from build123d import *

# Parameters (mm, degrees)
SALIENTE_EXTRUIR1_DEPTH = 5
CROQUIS4_R              = 3.275
CORTAR_EXTRUIR3_DEPTH   = 15
CROQUIS5_R              = 1.5
CORTAR_EXTRUIR4_DEPTH   = 10


with BuildPart() as part:
    # Croquis1 → Saliente-Extruir1 (new, symmetric)
    with BuildSketch(Plane.XY):
        Polygon((3, -8.75), (3, 13.75), (0, 13.75), (0, -13.75), (10, -13.75), (10, -8.75), align=None)
        Polygon((0, -13.75), (0, 13.75), (-3, 13.75), (-3, -8.75), (-10, -8.75), (-10, -13.75), align=None)
    extrude(amount=SALIENTE_EXTRUIR1_DEPTH, both=True)

    # Croquis4 → Cortar-Extruir3 (cut)
    with BuildSketch(Plane(origin=(3, 0, 0), x_dir=(0, 0, -1), z_dir=(1, 0, 0))):
        with Locations(Location((0, 3.55, 0), (0, 0, 90))):
            Circle(CROQUIS4_R)
    extrude(amount=-CORTAR_EXTRUIR3_DEPTH, mode=Mode.SUBTRACT)

    # Croquis5 → Cortar-Extruir4 (cut)
    with BuildSketch(Plane.XZ.offset(13.75)):
        with Locations((-6, 0)):
            Circle(CROQUIS5_R)
        with Locations(Location((6, 0, 0), (0, 0, 180))):
            Circle(CROQUIS5_R)
    extrude(amount=-CORTAR_EXTRUIR4_DEPTH, mode=Mode.SUBTRACT)


solid = part.part
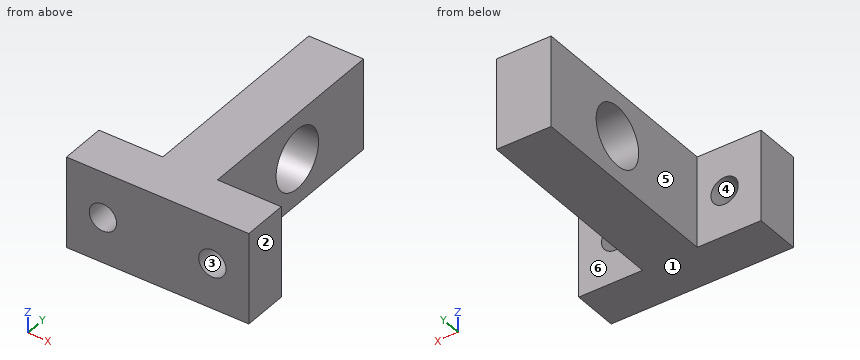
Here's how the part is built. I have some questions about the finished solid (model axes, mm). Face numbers are marked on the shaded views. A direction names the side the tool comes from. Coordinates: 2 decimals unless noted, no trailing zeros. Order: outer loops, then holes, each group sorted by start corner. A loop starts at its lowest first (then second) coordinate and runs counter-clockwise, first axis right, second up. Notation, with made-up numbers: M 64,71.25 L 78,71.25 A22 ccw 78,94.25 Z; hole C 37.5,-15 d8. An arc over 180 degrees is marked long. Answer as CSV lines item,"result". Start each with the question number.
1. For pin 1 (2.5 mm diameter, centred on x = -6, z = 0, fed in from -Y); pin 2 (5 mm diameter, centred on y = 0.5, z = -0.5, fed in from +X); pin 3 (5 mm diameter, centred on y = 0.5, z = 1, fed in from -X); pin 4 (3.5 mm diameter, centred on x = -7.5, z = 1.5, fed in from +Y), each with a flat end and sliding along its axis, tell me the tip position at first contact or that it passes through.
2. On a 3-axis mill with a long thin cutter (end or side, diameter ignored), from which of +Z, -Z, +X, -X, +Y, -Y can I reach the whole of each face in a straight line? I mean the marked faces 4, 5 and 6. Say none if no direction works.
3. We'd pull the mould along X, two halves only. Please class the marked faces 1, 2 and 3: released by +X, released by -X, zero draft, split by the parting line, or undercut.
4. I want a section at C-C, the plane z = -1. Write out the boundary of the cut face in (x, y).
5. I want a section at A-A, the plane x = -6. Write out the boundary of the cut face in (y, z).
6. I want a section at D-D, the plane x = -8. Write out the boundary of the cut face in (y, z), and give its area (3 significant figures).
7. I want a section at B-B, the plane y = 3.55. Write out the boundary of the cut face in (x, z) (3 decimals), and give its area (3 significant figures).
8. I need wall thicknesses on line 1 (Z direction, x = -0.05, y = 3.55) (3 decimals); line 2 (Z direction, x = -6, y = -11.15); line 3 (X direction, y = 1.5, z = -3.75). Which ranges of each line are inside material? Lowest first, please. Write a range as [from, to].
Recorded:
1,pin 1,"passes through"
1,pin 2,"stops at x = 3"
1,pin 3,"stops at x = -3"
1,pin 4,"stops at y = -8.75"
2,face 4,"+Y, -Y"
2,face 5,"+Z, -Z, -X, +Y"
2,face 6,"+Z, -Z, +X, +Y"
3,face 1,"zero draft"
3,face 2,"released by +X"
3,face 3,"undercut"
4,outline,"M -10,-13.75 L -7.12,-13.75 L -7.12,-8.75 L -10,-8.75 Z; M -4.88,-13.75 L 4.88,-13.75 L 4.88,-8.75 L 3,-8.75 L 3,0.43 L -3,0.43 L -3,-8.75 L -4.88,-8.75 Z; M -3,6.67 L 3,6.67 L 3,13.75 L -3,13.75 Z; M 7.12,-13.75 L 10,-13.75 L 10,-8.75 L 7.12,-8.75 Z"
5,outline,"M -13.75,-5 L -8.75,-5 L -8.75,-1.5 L -13.75,-1.5 Z; M -13.75,1.5 L -8.75,1.5 L -8.75,5 L -13.75,5 Z"
6,outline,"M -13.75,-5 L -8.75,-5 L -8.75,5 L -13.75,5 Z"
6,area,"50.0 mm2"
7,outline,"M -3,-5 L 3,-5 L 3,-3.275 L -3,-3.275 Z; M -3,3.275 L 3,3.275 L 3,5 L -3,5 Z"
7,area,"20.7 mm2"
8,line 1,"z = [-5, -3.275], [3.275, 5]"
8,line 2,"z = [-5, -1.5], [1.5, 5]"
8,line 3,"x = [-3, 3]"
